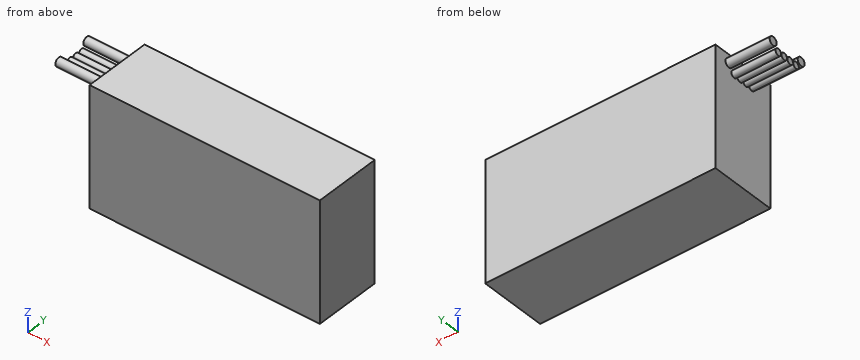
from build123d import *

# Parameters (mm, degrees)
SKETCH1_W           = 67.7
SKETCH1_H           = 19.6
BOSS_EXTRUDE1_DEPTH = 35.3
SKETCH3_R           = 1
SKETCH3_R_2         = 1.25
BOSS_EXTRUDE2_DEPTH = 13


with BuildPart() as part:
    # Sketch1 → Boss-Extrude1 (new body)
    with BuildSketch(Plane.XY):
        with Locations((33.85, 9.8)):
            Rectangle(SKETCH1_W, SKETCH1_H)
    extrude(amount=BOSS_EXTRUDE1_DEPTH)

    # Sketch3 → Boss-Extrude2 (add)
    with BuildSketch(Plane.ZY):
        with Locations(Location((30.7, 12.95, 0), (0, 0, 180))):
            Circle(SKETCH3_R)
        with Locations(Location((30.7, 10.85, 0), (0, 0, 180))):
            Circle(SKETCH3_R)
        with Locations(Location((30.7, 8.75, 0), (0, 0, 180))):
            Circle(SKETCH3_R)
        with Locations(Location((32.8, 4.8, 0), (0, 0, 180))):
            Circle(SKETCH3_R_2)
        with Locations(Location((32.8, 14.8, 0), (0, 0, 180))):
            Circle(SKETCH3_R_2)
        with Locations(Location((30.7, 6.65, 0), (0, 0, 180))):
            Circle(SKETCH3_R)
    extrude(amount=BOSS_EXTRUDE2_DEPTH)


solid = part.part
Part model, mm, in its own coordinate system. Coordinates: 2 decimals unless noted, no trailing zeros. Loops run counter-clockwise (first coordinate to the right, second up) from the corner with the lowest first, then second, coordinate; pieces in that order, holes last. Notation, with made-up numbers: (62, 20.5) -> (76, 20.5) arc R25 cw to (76, 58.5) -> close; hole circle Ø8 at (64, 40). An arc over 180 degrees is marked (long way). Use a Markdown table: item, result. Add a question column.
Item 1: Band-saw the part on D-D on z = 2. Write the cut outline in (x, y), plus the area to 3 significant figures.
Item 2: Band-saw the part on C-C on y = 4.8. Write the cut outline in (x, z).
Item 3: Flat gauge pin, fed straight in: P1, Ø1.5, axis at y = 8.5, z = 22.5, coming from the -X side. Where does the tip first touch, or does it go through?
Item 4: Probe probe 1 along X at (y, z) = (5.25, 15.5). List the from-to ranges inside material, lowest first.
Item 5: Band-saw the part on B-B on z = 32.8. Write the cut outline in (x, y), plus the area to 3 significant figures.
Item 6: Band-saw the part on A-A on y = 8.75. Write the cut outline in (x, z).
Geometry says:
| question | item | result |
|---|---|---|
| 1 | outline | (0, 0) -> (67.7, 0) -> (67.7, 19.6) -> (0, 19.6) -> close |
| 1 | area | 1,330 mm² |
| 2 | outline | (-13, 31.55) -> (0, 31.55) -> (0, 0) -> (67.7, 0) -> (67.7, 35.3) -> (0, 35.3) -> (0, 34.05) -> (-13, 34.05) -> close |
| 3 | P1 | x = 0 |
| 4 | probe 1 | 0 to 67.7 |
| 5 | outline | (-13, 3.55) -> (0, 3.55) -> (0, 0) -> (67.7, 0) -> (67.7, 19.6) -> (0, 19.6) -> (0, 16.05) -> (-13, 16.05) -> (-13, 13.55) -> (0, 13.55) -> (0, 6.05) -> (-13, 6.05) -> close |
| 5 | area | 1,390 mm² |
| 6 | outline | (-13, 29.7) -> (0, 29.7) -> (0, 0) -> (67.7, 0) -> (67.7, 35.3) -> (0, 35.3) -> (0, 31.7) -> (-13, 31.7) -> close |
